The figure shows three views and two pictorial views of one solid part (mm, origin at its lowest corner). Answer the questions. Coordinates: 2 decimals unless noted, no trailing zeros. Order: outer loops, then holes, each group sorted by start corner. A loop starts at its lowest first (then second) coordinate and runs counter-clockwise, first axis right, second up. Notation, with made-up numbers: M -3.5,-5 L 14.5,-5 A21 cw 14.5,16 Z; hole C -15,74.25 d11. An arc over 180 degrees is marked long. Write item = value, one per line. Start each with the question number.
Q1. Determine the mould class of the marked faces 1, 2 and 3 for opening direction Z: released by +Z, released by -Z, zero draft, split by the parting line, or undercut.
Q2. Find section C-C on z = 59. Give the vertices of the cut face in (x, y), and give its area (3 significant figures).
Q3. Find section A-A on x = 75. Give the vertices of the cut face in (y, z), and give its area (3 significant figures).
Q4. Straight lines are drawn through the part: line 1 along X through (y, z) = (8.5, 75); line 2 along X through (y, z) = (2.75, 87) (1 decimal); line 3 along X through (y, z) = (13.5, 52) (1 decimal). For each, find the intervals that lie inside material, in ascending order.
Q5. Each of these flat-tipped pins is pushed along its axis until it touches: P1, Ø8, axis at y = 3, z = 82, coming from the +X side; P2, Ø8, axis at x = 40.5, y = 13.5, coming from the -Z side; P3, Ø4, axis at y = 14.5, z = 97.5, coming from the -X side. Where does it stop, or does it pass through?
Q6. Find section D-D on y = 11.75. Give the vertices of the cut face in (x, z) (1 decimal).
Q7. Find section B-B on z = 75. Give the vertices of the cut face in (x, y).
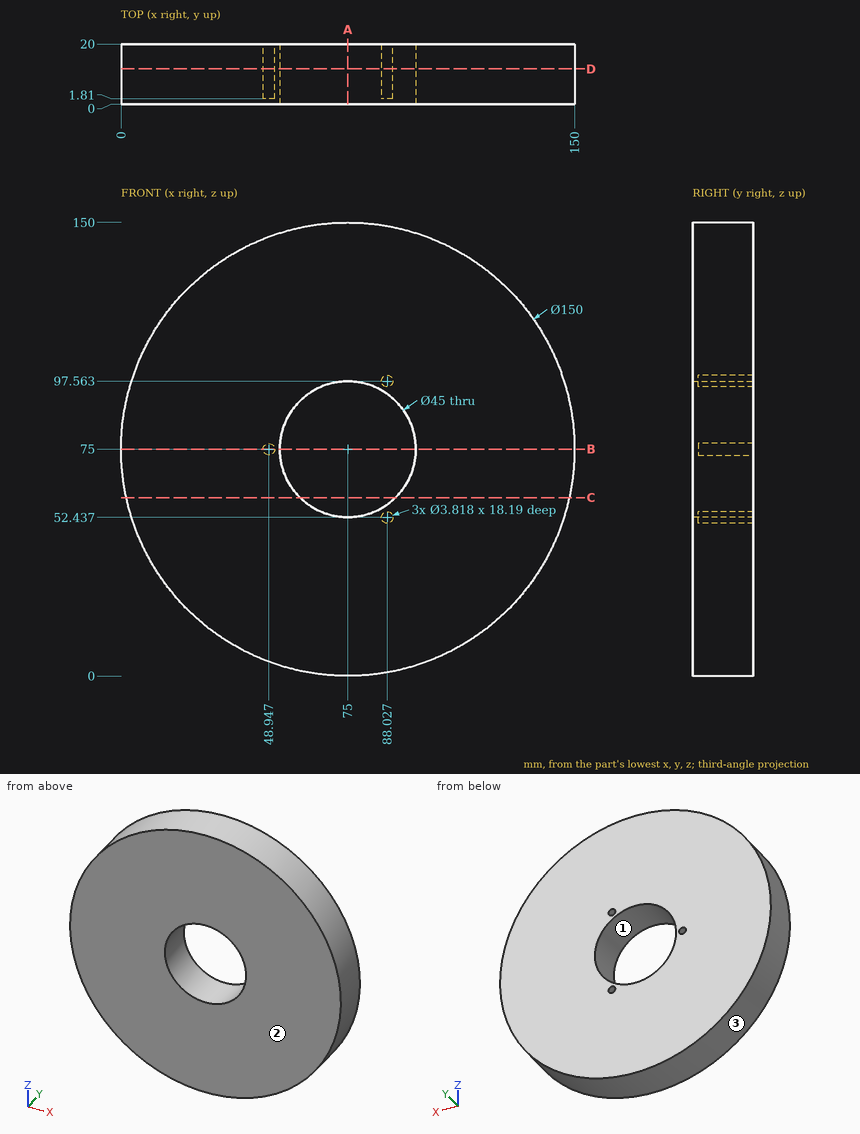
Findings below:
q1.face_1 = undercut
q1.face_2 = zero draft
q1.face_3 = split by the parting line
q2.outline = M 1.73,0 L 59.18,0 L 59.18,20 L 1.73,20 Z; M 90.82,0 L 148.27,0 L 148.27,20 L 90.82,20 Z
q2.area = 2,300 mm^2
q3.outline = M 0,0 L 20,0 L 20,52.5 L 0,52.5 Z; M 0,97.5 L 20,97.5 L 20,150 L 0,150 Z
q3.area = 2,100 mm^2
q4.line_1 = 0 to 47.04, 50.86 to 52.5, 97.5 to 150
q4.line_2 = 1 to 56, 94 to 149
q4.line_3 = 3.6 to 86.2, 89.9 to 146.4
q5.P1 = 149.94
q5.P2 = 6.48
q5.P3 = 2.86
q6.outline = C 75,75 d150; hole C 48.9,75 d3.8; hole C 75,75 d45; hole C 88,52.4 d3.8; hole C 88,97.6 d3.8
q7.outline = M 0,0 L 52.5,0 L 52.5,20 L 50.86,20 L 50.86,1.81 L 47.04,1.81 L 47.04,20 L 0,20 Z; M 97.5,0 L 150,0 L 150,20 L 97.5,20 Z
